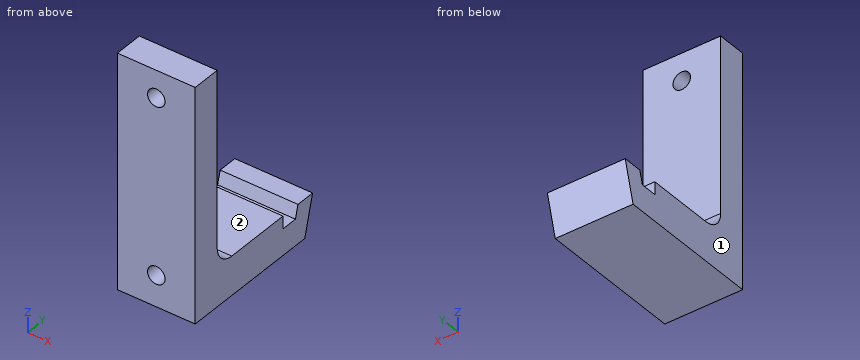
```python
from build123d import *

# Parameters (mm, degrees)
BOSS_EXTRUDE1_DEPTH = 4
FILLET1_R           = 2
SKETCH2_R           = 0.9
CUT_EXTRUDE1_DEPTH  = 4


with BuildPart() as part:
    # Sketch1 → Boss-Extrude1 (new, symmetric)
    with BuildSketch(Plane(origin=(0, 0, 0), x_dir=(0, 0, -1), z_dir=(1, 0, 0))):
        Polygon((0, 3), (20, 3), (20, 12), (21.3, 12), (21.3, 13.7), (20, 14.04833395), (20, 16.04833395), (24, 14.97653718), (24, 0), (0, 0), align=None)
    extrude(amount=BOSS_EXTRUDE1_DEPTH, both=True)

    # Fillet1
    fillet1_edges = [part.edges().sort_by_distance(p)[0] for p in [
        (0, 3, -20),
    ]]
    fillet(fillet1_edges, radius=FILLET1_R)

    # Sketch2 → Cut-Extrude1 (cut)
    with BuildSketch(Plane.XZ):
        with Locations(Location((0, -20.8, 0), (0, 0, 270))):
            Circle(SKETCH2_R)
        with Locations(Location((0, -2.8, 0), (0, 0, 270))):
            Circle(SKETCH2_R)
    extrude(amount=-CUT_EXTRUDE1_DEPTH, mode=Mode.SUBTRACT)


solid = part.part
```
The listing builds one solid part. Answer for the finished solid, in the listing's coordinates (mm). Face numbers are marked on the shaded views. A direction names the side the tool comes from. Give positions to 0.01 mm unless a question says otherwise; leave off trailing zeros. Order: outer loops, then holes, each group sorted by start corner. A loop starts at its lowest first (then second) coordinate and runs counter-clockwise, first axis right, second up.
Item 1: Find the intervals of material crossed by probe 1 along X at (y, z) = (1.9, -2.8); probe 2 along Z at (x, y) = (-0.75, 8.5); probe 3 along Y at (x, z) = (1, -7.5), in increasing order.
From the geometry:
probe 1: x = -4 to -0.9, 0.9 to 4
probe 2: z = -24 to -20
probe 3: y = 0 to 3
Item 2: The part is cut by section A-A, the plane z = -2.8. Give the vertices of the cut face in (x, y), and give its area (3 significant figures).
From the geometry:
outline: (-4, 0) - (-0.9, 0) - (-0.9, 3) - (-4, 3) - close; (0.9, 0) - (4, 0) - (4, 3) - (0.9, 3) - close
area: 18.6 mm2
Item 3: The part is cut by section D-D, the plane y = 9.25. Give the vertices of the cut face in (x, z).
From the geometry:
outline: (-4, -24) - (4, -24) - (4, -20) - (-4, -20) - close
Item 4: The part is cut by section C-C, the plane x = -1.5. Give the vertices of the cut face in (y, z).
From the geometry:
outline: (0, -24) - (14.98, -24) - (16.05, -20) - (14.05, -20) - (13.7, -21.3) - (12, -21.3) - (12, -20) - (5, -20) arc R2 cw to (3, -18) - (3, 0) - (0, 0) - close
Item 5: The part is cut by section B-B, the plane x = 0. Give the vertices of the cut face in (y, z).
From the geometry:
outline: (0, -24) - (14.98, -24) - (16.05, -20) - (14.05, -20) - (13.7, -21.3) - (12, -21.3) - (12, -20) - (5, -20) arc R2 cw to (3, -18) - (3, -3.7) - (0, -3.7) - (0, -19.9) - (4, -19.9) - (4, -21.7) - (0, -21.7) - close; (0, -1.9) - (3, -1.9) - (3, 0) - (0, 0) - close
Item 6: Which of the six approach directions +Z, -Z, +X, -X, +Y, -Y give full straight-line access (tool end or side, diameter ignored) to the marked faces 1 and 2?
From the geometry:
face 1: +Z, -Z, -X, +Y, -Y
face 2: +Z, +X, -X, +Y
Item 7: Given pin 1 Ø3.5 at (x, y) = (-1, 7.5) entering from +Z; pin 2 Ø0.7 at (x, z) = (-1, -20.5) entering from +Y; pin 3 Ø3 at (x, z) = (-2.5, -15) entering from +Y, each flat-ended and moving along its own axis, determine where each tip first touches the part or whether it passes through.
From the geometry:
pin 1: stops at z = -20
pin 2: stops at y = 16.01
pin 3: stops at y = 3
